Work out the finished part from the listing and answer in its coordinate system (mm). Face numbers are marked on the shaded views. A direction names the side the tool comes from. Coordinates: 2 decimals unless noted, no trailing zeros. Order: outer loops, then holes, each group sorted by start corner. A loop starts at its lowest first (then second) coordinate and runs counter-clockwise, first axis right, second up. Notation, with made-up numbers: M 87.25,-19 L 116.25,-19 A27 cw 116.25,9 Z; hole C -36,-38 d8. An arc over 180 degrees is marked long. Use a Markdown table: item, result.
from build123d import *

# Parameters (mm, degrees)
BOSS_EXTRUDE1_DEPTH       = 7.62
F_6_32_TAPPED_HOLE1_D     = 2.7051
F_6_32_TAPPED_HOLE1_DEPTH = 0.635
CUT_EXTRUDE1_REACH        = 9.62
SKETCH6_R                 = 2.159
CUT_EXTRUDE6_DEPTH        = 8.62
SKETCH27_W                = 5.344661664
SKETCH27_H                = 4.789513508
BOSS_EXTRUDE2_DEPTH       = 0.0254


with BuildPart() as part:
    # Sketch1 → Boss-Extrude1 (new body)
    with BuildSketch(Plane.XY):
        Polygon((-3.353873239, 6.85218662), (-3.353873239, -2.29181338), (4.266126761, -2.29181338), (4.266126761, 6.85218662), (3.631126761, 6.85218662), (3.631126761, -1.52981338), (-2.718873239, -1.52981338), (-2.718873239, 6.85218662), align=None)
    extrude(amount=BOSS_EXTRUDE1_DEPTH)

    # #6-32 Tapped Hole1
    with Locations(Plane.ZY.offset(3.353873239)):
        with Locations((3.81, 4.05818662)):
            Hole(F_6_32_TAPPED_HOLE1_D / 2, depth=F_6_32_TAPPED_HOLE1_DEPTH)

    # Sketch6 → Cut-Extrude1 (cut, up to next)
    with BuildSketch(Plane(origin=(4.266126761, 0, 0), x_dir=(0, 0, -1), z_dir=(1, 0, 0)), mode=Mode.PRIVATE) as cut_extrude1_sk1:
        with Locations((-3.81, 4.05818662)):
            Circle(SKETCH6_R)
    cut_extrude1_tool1 = extrude(cut_extrude1_sk1.sketch, amount=-CUT_EXTRUDE1_REACH, mode=Mode.PRIVATE) & part.part
    add(cut_extrude1_tool1.solids().sort_by_distance((4.266127, 4.058187, 3.81))[0], mode=Mode.SUBTRACT)

    # Sketch26 → Cut-Extrude6 (cut, through all)
    with BuildSketch(Plane(origin=(4.266126761, 0, 0), x_dir=(0, 0, -1), z_dir=(1, 0, 0))):
        with BuildLine():
            add(Edge.make_bspline(
                [(0, 0), (0, 6.85218662), (-3.81, 6.85218662)],
                knots=[4.71238898, 4.71238898, 4.71238898, 6.283185307, 6.283185307, 6.283185307], degree=2, weights=[1, 0.707106781, 1]))
            Line((0, 0), (0, 6.85218662))
            Line((0, 6.85218662), (-3.81, 6.85218662))
        make_face()
        with BuildLine():
            add(Edge.make_bspline(
                [(-3.81, 6.85218662), (-7.62, 6.85218662), (-7.62, 0)],
                knots=[6.283185307, 6.283185307, 6.283185307, 7.853981634, 7.853981634, 7.853981634], degree=2, weights=[1, 0.707106781, 1]))
            Line((-3.81, 6.85218662), (-7.62, 6.85218662))
            Line((-7.62, 6.85218662), (-7.62, 0))
        make_face()
    extrude(amount=-CUT_EXTRUDE6_DEPTH, mode=Mode.SUBTRACT)

    # Sketch27 → Boss-Extrude2 (add)
    with BuildSketch(Plane.XZ.offset(2.29181338)):
        with Locations((0.586749856, 3.842655774)):
            Rectangle(SKETCH27_W, SKETCH27_H)
    extrude(amount=BOSS_EXTRUDE2_DEPTH)


solid = part.part
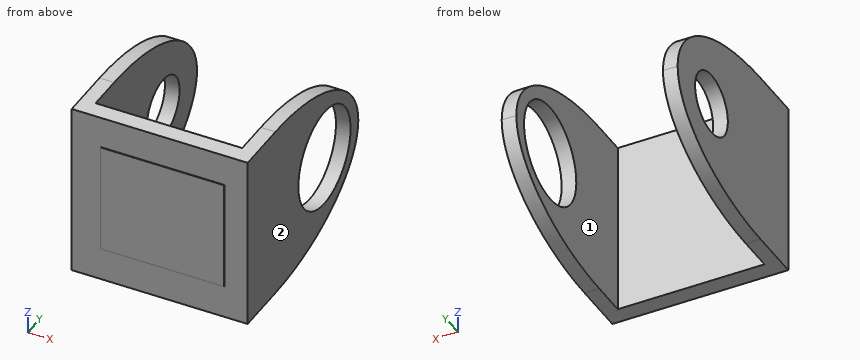
1. Section C-C on y = 3 is taken. Give the number of separate pieces and of enclosed holes in the cut face, then the cut area to 3 significant figures.
Answers below:
| item | result |
|---|---|
| separate pieces | 4 |
| enclosed holes | 0 |
| area | 5.24 mm² |
2. Section A-A on y = -0.5 is taken. Determine the outline of the cut face in (x, z).
Answers below:
| item | result |
|---|---|
| outline | M -3.35,0 L -2.72,0 L -2.72,7.62 L -3.35,7.62 Z; M 3.63,0 L 4.27,0 L 4.27,7.62 L 3.63,7.62 Z |
3. A flat-ended cylindrical pin translates along its axis: P1, Ø3, axis at x = 3, y = 4.5, coming from the -Z side. Find the tip coordinate at first contact, or state that the pin passes through.
Answers below:
| item | result |
|---|---|
| P1 | z = 0.42 |
4. Find the intervals of material crossed by probe 1 along X at (y, z) = (2.5, 6.75); probe 2 along Y at (x, z) = (4, 3.81); probe 3 along Y at (x, z) = (-2.9, 3.81), in increasing order.
Answers below:
| item | result |
|---|---|
| probe 1 | -3.35 to -2.72, 3.63 to 4.27 |
| probe 2 | -2.29 to 1.9, 6.22 to 6.85 |
| probe 3 | -2.29 to 2.71, 5.41 to 6.85 |
5. For the marked faces 1 and 2, determine the directions among +Z, -Z, +X, -X, +Y, -Y from which every point of the face is accessible in a straight line to the end or side of a thin tool.
Answers below:
| item | result |
|---|---|
| face 1 | +Z, -Z, +Y |
| face 2 | +Z, -Z, +X, +Y, -Y |
